Work out the finished part from the listing and answer in its coordinate system (mm). Give positions to 0.01 mm unless a question says otherwise; leave off trailing zeros. Write each loop counter-clockwise with the first axis right and the second up, starting at its lowest first coordinate (ties: lowest second). Pieces come first, ordered by that corner, then holes. Notation, with made-up numbers: (50.5, -34.75) -> (67.5, -34.75) arc R35 ccw to (67.5, 1.25) -> close; hole circle Ø9 at (-15.75, -39.5). An arc over 180 degrees is marked (long way). Use a Markdown table: item, result. Add a question column.
Q1. Section C-C, the plane z = 31.75 is taken. Give the vertices of the cut face in (x, y).
Q2. Section B-B, the plane y = 1.1 is taken. State how many separate pieces and enclosed holes the cut face has, plus the area to 3 significant figures.
Q3. Section D-D, the plane x = 21.59 is taken. Give the vertices of the cut face in (y, z), plus the area to 3 significant figures.
Q4. Consider line 1 (X direction, y = 1.35, z = 15.5); line 2 (Z direction, x = -21, y = 0.5); line 3 (X direction, y = -0.35, z = 31.75). Determine where each line is inside the solid, lowest interval first.
Q5. Each of these flat-tipped pins is pushed along its axis until it touches: pin 1 Ø5.5 at (x, z) = (0, 31.75) entering from -Y; pin 2 Ø1 at (y, z) = (-1, 8.5) entering from -X. Where does it stop, or does it pass through?
Q6. Section A-A, the plane x = 0 is taken. Give the vertices of the cut face in (y, z), plus the area to 3 significant figures.
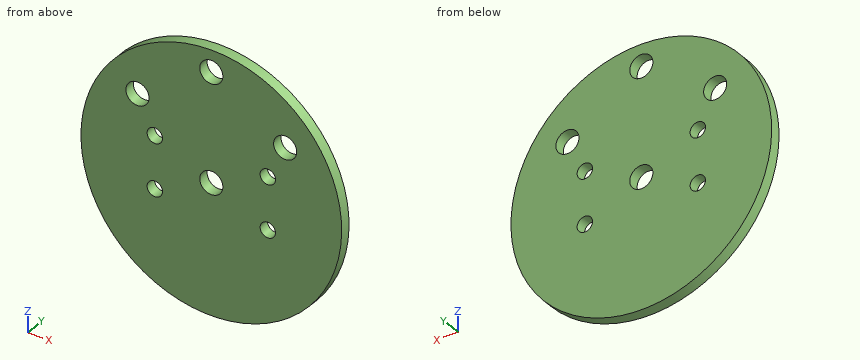
from build123d import *

# Parameters (mm, degrees)
SKETCH1_R               = 38.1
BOSS_EXTRUDE1_DEPTH     = 1.5875
F_1_4_CLEARANCE_HOLE1_D = 6.7564
F_1_4_CLEARANCE_HOLE2_D = 6.7564
F_1_4_CLEARANCE_HOLE3_D = 6.7564
F_8_CLEARANCE_HOLE1_D   = 4.4958


with BuildPart() as part:
    # Sketch1 → Boss-Extrude1 (new, symmetric)
    with BuildSketch(Plane(origin=(0, 0, 0), x_dir=(1, 0, 0), z_dir=(0, 1, 0))):
        with Locations(Location((0, 0, 0), (0, 0, 270))):
            Circle(SKETCH1_R)
    extrude(amount=BOSS_EXTRUDE1_DEPTH, both=True)

    # 1/4 Clearance Hole1 (through all)
    with Locations(Plane(origin=(0, 1.5875, 0), x_dir=(1, 0, 0), z_dir=(0, 1, 0))):
        with Locations((-21.59, -17.810706314), (21.59, -17.810706314)):
            Hole(F_1_4_CLEARANCE_HOLE1_D / 2)

    # 1/4 Clearance Hole2 (through all)
    with Locations(Plane(origin=(0, 1.5875, 0), x_dir=(1, 0, 0), z_dir=(0, 1, 0))):
        with Locations((0, 0)):
            Hole(F_1_4_CLEARANCE_HOLE2_D / 2)

    # 1/4 Clearance Hole3 (through all)
    with Locations(Plane(origin=(0, 1.5875, 0), x_dir=(1, 0, 0), z_dir=(0, 1, 0))):
        with Locations((0, -31.75)):
            Hole(F_1_4_CLEARANCE_HOLE3_D / 2)

    # #8 Clearance Hole1 (through all)
    with Locations(Plane(origin=(0, 1.5875, 0), x_dir=(1, 0, 0), z_dir=(0, 1, 0))):
        with Locations((-16.51, 7.62), (-16.51, -7.62), (16.51, -7.62), (16.51, 7.62)):
            Hole(F_8_CLEARANCE_HOLE1_D / 2)


solid = part.part
Result set:
| question | item | result |
|---|---|---|
| 1 | outline | (-21.06, -1.59) -> (-3.38, -1.59) -> (-3.38, 1.59) -> (-21.06, 1.59) -> close; (3.38, -1.59) -> (21.06, -1.59) -> (21.06, 1.59) -> (3.38, 1.59) -> close |
| 2 | separate pieces | 1 |
| 2 | enclosed holes | 8 |
| 2 | area | 4,350 mm2 |
| 3 | outline | (-1.59, -31.39) -> (1.59, -31.39) -> (1.59, 14.43) -> (-1.59, 14.43) -> close; (-1.59, 21.19) -> (1.59, 21.19) -> (1.59, 31.39) -> (-1.59, 31.39) -> close |
| 3 | area | 178 mm2 |
| 4 | line 1 | x = -34.8 to -24.05, -19.13 to 19.13, 24.05 to 34.8 |
| 4 | line 2 | z = -31.79 to 14.48, 21.14 to 31.79 |
| 4 | line 3 | x = -21.06 to -3.38, 3.38 to 21.06 |
| 5 | pin 1 | passes through |
| 5 | pin 2 | stops at x = -37.25 |
| 6 | outline | (-1.59, -38.1) -> (1.59, -38.1) -> (1.59, -3.38) -> (-1.59, -3.38) -> close; (-1.59, 3.38) -> (1.59, 3.38) -> (1.59, 28.37) -> (-1.59, 28.37) -> close; (-1.59, 35.13) -> (1.59, 35.13) -> (1.59, 38.1) -> (-1.59, 38.1) -> close |
| 6 | area | 199 mm2 |
